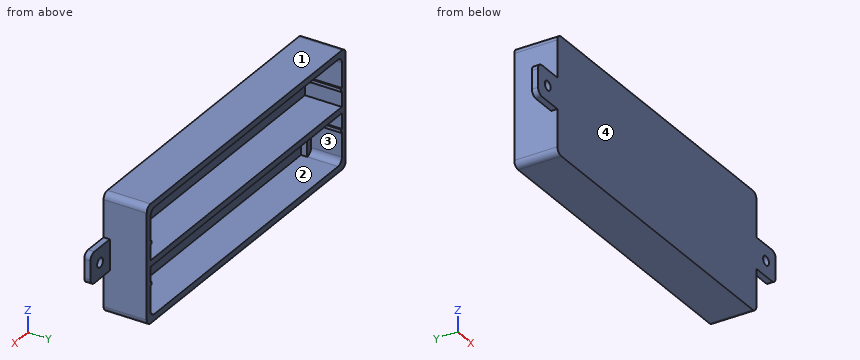
Autodesk Inventor part; units mm, degrees
ref_plane "YZ Plane" through (0, 0, 0) normal (1, 0, 0) x (0, 1, 0)
ref_plane "XZ Plane" through (0, 0, 0) normal (0, 1, 0) x (-1, 0, 0)
ref_plane "XY Plane" through (0, 0, 0) normal (0, 0, 1) x (1, 0, 0)
sketch "Sketch1" plane through (0, 0, 0) normal (0, 1, 0) x (-1, 0, 0)
  line L0 (0, 0) -> (-103, 0)
  line L1 (-103, 0) -> (-103, -38)
  line L2 (-103, -38) -> (0, -38)
  line L3 (0, -38) -> (0, 0)
  dimension "d0" = 103
  dimension "d1" = 38
extrude "Extrusion1" add sketch "Sketch1" along normal blind 2
sketch "Sketch2" plane through (0, 2, 0) normal (0, 1, 0) x (1, 0, 0)
  line L0 (2, 2) -> (101, 2)
  line L1 (101, 2) -> (101, 18)
  line L2 (101, 18) -> (2, 18)
  line L3 (2, 18) -> (2, 2)
  line L4 (2, 20) -> (101, 20)
  line L5 (101, 20) -> (101, 36)
  line L6 (101, 36) -> (2, 36)
  line L7 (2, 36) -> (2, 20)
  line L8 (0, 0) -> (2, 0)
  line L9 (2, 0) -> (2, 2)
  line L10 (2, 2) -> (0, 2)
  line L11 (0, 2) -> (0, 0)
  line L12 (103, 38) -> (0, 38)
  line L13 (0, 38) -> (2, 38)
  line L14 (2, 38) -> (2, 36)
  line L15 (2, 36) -> (0, 36)
  line L16 (0, 36) -> (0, 38)
  line L17 (103, 0) -> (103, 38)
  line L18 (0, 0) -> (103, 0)
  line L19 (103, 0) -> (103, 38)
  line L20 (103, 38) -> (0, 38)
  line L21 (0, 38) -> (0, 0)
  dimension "d4" = 99
  dimension "d5" = 16
  dimension "d6" = 99
  dimension "d7" = 16
  dimension "d8" = 2
  dimension "d9" = 2
  dimension "d10" = 2
  dimension "d11" = 2
extrude "Extrusion2" add sketch "Sketch2" along normal blind 12
sketch "Sketch3" plane through (101, 2, -18) normal (-1, 0, 0) x (0, 0, 1)
  line L0 (18, 12) -> (-20, 12)
  line L1 (5, 12) -> (6, 12)
  line L2 (6, 12) -> (6, 0)
  line L3 (6, 0) -> (5, 0)
  line L4 (5, 0) -> (5, 12)
  line L5 (0, 12) -> (5, 12)
  line L6 (5, 12) -> (5, 0)
  line L7 (5, 0) -> (0, 0)
  line L8 (0, 0) -> (0, 12)
  point P0 (18, -2)
  dimension "d14" = 1
  dimension "d15" = 12
  dimension "d16" = 5
  dimension "d17" = 12
extrude "Extrusion3" add sketch "Sketch3" along normal blind 0.5 contours L2 L3 L4 L0
sketch "Sketch4" plane through (2, 2, -2) normal (1, 0, 0) x (0, 0, -1)
  line L0 (16, 12) -> (11, 12)
  line L1 (11, 12) -> (11, 0)
  line L2 (11, 0) -> (16, 0)
  line L3 (16, 0) -> (16, 12)
  line L4 (11, 12) -> (10, 12)
  line L5 (10, 12) -> (10, 0)
  line L6 (10, 0) -> (11, 0)
  line L7 (11, 0) -> (11, 12)
  point P0 (-2, -2)
  point P1 (11, 0)
  dimension "d20" = 5
  dimension "d21" = 12
  dimension "d22" = 1
  dimension "d23" = 12
extrude "Extrusion4" add sketch "Sketch4" along normal blind 0.5 contours L1 L6 L5 L4
sketch "Sketch5" plane through (2, 2, -20) normal (1, 0, 0) x (0, 0, -1)
  line L0 (0, 12) -> (5, 12)
  line L1 (5, 12) -> (5, 0)
  line L2 (5, 0) -> (0, 0)
  line L3 (0, 0) -> (0, 12)
  line L4 (5, 12) -> (6, 12)
  line L5 (6, 12) -> (6, 0)
  line L6 (6, 0) -> (5, 0)
  line L7 (5, 0) -> (5, 12)
  point P0 (-20, -2)
  point P1 (5, 0)
  dimension "d26" = 5
  dimension "d27" = 12
  dimension "d28" = 1
  dimension "d29" = 12
extrude "Extrusion5" add sketch "Sketch5" along normal blind 0.5 contours L4 L5 L6 L1
sketch "Sketch6" plane through (101, 2, -36) normal (-1, 0, 0) x (0, 0, 1)
  line L0 (16, 12) -> (11, 12)
  line L1 (11, 12) -> (11, 0)
  line L2 (11, 0) -> (16, 0)
  line L3 (16, 0) -> (16, 12)
  line L4 (11, 12) -> (10, 12)
  line L5 (10, 12) -> (10, 0)
  line L6 (10, 0) -> (11, 0)
  line L7 (11, 0) -> (11, 12)
  point P0 (36, -2)
  point P1 (11, 0)
  dimension "d32" = 5
  dimension "d33" = 12
  dimension "d34" = 1
  dimension "d35" = 12
extrude "Extrusion6" add sketch "Sketch6" along normal blind 0.5 contours L1 L6 L5 L4
sketch "Sketch7" plane through (103, 0, 0) normal (1, 0, 0) x (0, 0, -1)
  line L0 (14, 0) -> (24, 0)
  line L1 (24, 0) -> (24, 2)
  line L2 (24, 2) -> (14, 2)
  line L3 (14, 2) -> (14, 0)
  line L4 (0, 0) -> (38, 0)
  point P0 (19, 0)
  dimension "d38" = 10
  dimension "d39" = 2
extrude "Extrusion7" add sketch "Sketch7" along normal blind 10
sketch "Sketch8" plane through (103, 2, -14) normal (0, 1, 0) x (1, 0, 0)
  line L0 (10, 10) -> (10, 0)
  line L1 (10, 5) -> (0, 5)
  line L2 (0, -14) -> (0, 24)
  circle A0 centre (5, 5) radius 1.5
  point P0 (-103, -14)
  dimension "d42" = 3
extrude "Extrusion8" cut sketch "Sketch8" against normal blind 2
sketch "Sketch9" plane through (0, 0, -38) normal (-1, 0, 0) x (0, 0, 1)
  line L0 (24, 0) -> (14, 0)
  line L1 (14, 0) -> (14, 2)
  line L2 (14, 2) -> (24, 2)
  line L3 (24, 2) -> (24, 0)
  line L4 (0, 0) -> (38, 0)
  point P0 (19, 0)
  dimension "d45" = 10
  dimension "d46" = 2
extrude "Extrusion9" add sketch "Sketch9" along normal blind 10
sketch "Sketch10" plane through (0, 2, -14) normal (0, 1, 0) x (1, 0, 0)
  line L0 (-10, 10) -> (-10, 0)
  line L1 (-10, 5) -> (0, 5)
  line L2 (0, 24) -> (0, -14)
  circle A0 centre (-5, 5) radius 1.5
  dimension "d49" = 3
extrude "Extrusion10" cut sketch "Sketch10" against normal blind 2
fillet "Fillet1" radius 2 12 edges at (0, 7, 0) (103, 7, 0) (103, 7, -38) (113, 1, -14) (113, 1, -24) (0, 7, -38) (-10, 1, -24) (-10, 1, -14) (2, 8, -36) (101, 8, -36) (101, 8, -2) (2, 8, -2)
sketch "Sketch11" plane through (0, 2, 0) normal (0, 1, 0) x (1, 0, 0)
  line L0 (101, 36) -> (99, 36)
  line L1 (99, 36) -> (99, 29.4)
  line L2 (99, 29.4) -> (101, 29.4)
  line L3 (101, 29.4) -> (101, 36)
  line L4 (2, 36) -> (4, 36)
  line L5 (4, 36) -> (4, 29.4)
  line L6 (4, 29.4) -> (2, 29.4)
  line L7 (2, 29.4) -> (2, 36)
  line L8 (2, 2) -> (4, 2)
  line L9 (4, 2) -> (4, 8.6)
  line L10 (4, 8.6) -> (2, 8.6)
  line L11 (2, 8.6) -> (2, 2)
  line L12 (101, 2) -> (99, 2)
  line L13 (99, 2) -> (99, 8.6)
  line L14 (99, 8.6) -> (101, 8.6)
  line L15 (101, 8.6) -> (101, 2)
  point P0 (0, 0)
  dimension "d53" = 2
  dimension "d54" = 6.6
  dimension "d55" = 2
  dimension "d56" = 6.6
  dimension "d57" = 2
  dimension "d58" = 6.6
  dimension "d59" = 2
  dimension "d60" = 6.6
extrude "Extrusion11" add sketch "Sketch11" along normal blind 2
properties part number "power_strip"
Verification items for the finished model (mm, model axes). Face numbers are marked on the shaded views. A direction names the side the tool comes from. Give positions to 0.01 mm unless a question says otherwise; leave off trailing zeros. Loops run counter-clockwise (first coordinate to the right, second up) from the corner with the lowest first, then second, coordinate; pieces in that order, holes last.
1) Depth check by flat-ended pin: pin 1 Ø5 at (x, z) = (31, -11) entering from +Y; pin 2 Ø2 at (y, z) = (11.5, -30.5) entering from -X; pin 3 Ø1.6 at (x, z) = (99.5, -33.5) entering from +Y. Enter the tip coordinate at first touch or a pass-through.
2) Thickness scan on line 1 along Z through (x, y) = (18, 8); line 2 along X through (y, z) = (0.9, -19); line 3 along X through (y, z) = (12, -24). Record the ranges inside material, lowest first.
3) Draft check along X on the marked faces 3 and 4. Enter one of: pulls with the +X half, pulls with the -X half, needs draft (parallel to the pull), parting line crosses it, or undercut.
4) Sectioned sample at B-B, the plane x = 83. Enter the section's corners in (y, z), then the cut area to 3 significant figures.
5) Set-up check for the marked faces 1 and 2: record each of +Z, -Z, +X, -X, +Y, -Y from which the full face is reachable in a straight line by a thin tool's end or side.
6) Sectioned sample at C-C, the plane y = 12. Count the separate pieces of the cut face and the enclosed holes in it, then the cut area to 3 significant figures.
7) Sectioned sample at A-A, the plane x = 108. Enter the section's corners in (y, z).
Answers:
1. pin 1: stops at y = 2
1. pin 2: stops at x = 0
1. pin 3: stops at y = 4
2. line 1: z = -38 to -36, -20 to -18, -2 to 0
2. line 2: x = -10 to -6.5, -3.5 to 106.5, 109.5 to 113
2. line 3: x = 0 to 2, 101 to 103
3. face 3: undercut
3. face 4: needs draft
4. outline: (0, -38) - (14, -38) - (14, -36) - (2, -36) - (2, -20) - (14, -20) - (14, -18) - (2, -18) - (2, -2) - (14, -2) - (14, 0) - (0, 0) - close
4. area: 148 mm2
5. face 1: +Z, +X, -X, +Y, -Y
5. face 2: +Y
6. separate pieces: 1
6. enclosed holes: 2
6. area: 748 mm2
7. outline: (0, -24) - (2, -24) - (2, -20.5) - (0, -20.5) - close; (0, -17.5) - (2, -17.5) - (2, -14) - (0, -14) - close
